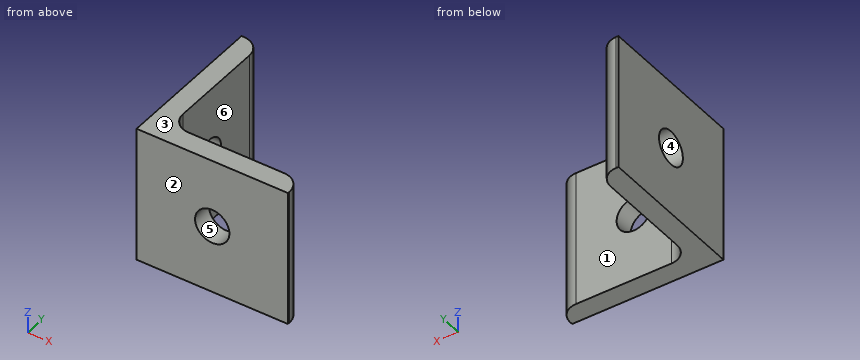
from build123d import *

# Parameters (mm, degrees)
BOSS_EXTRUDE1_DEPTH = 13.5
SKETCH4_R           = 3.4036
CUT_EXTRUDE3_DEPTH  = 10
SKETCH5_R           = 3.4036
CUT_EXTRUDE4_DEPTH  = 10


with BuildPart() as part:
    # Sketch1 → Boss-Extrude1 (new body, symmetric)
    with BuildSketch(Plane.XY):
        with BuildLine():
            Line((0, 0), (30, 0))
            Line((30, 0), (30, 0.5))
            ThreePointArc((30, 0.5), (28.974873734, 2.974873734), (26.5, 4))
            Line((26.5, 4), (7.5, 4))
            ThreePointArc((7.5, 4), (5.025126266, 5.025126266), (4, 7.5))
            Line((4, 7.5), (4, 26.5))
            ThreePointArc((4, 26.5), (2.974873734, 28.974873734), (0.5, 30))
            Line((0.5, 30), (0, 30))
            Line((0, 30), (0, 0))
        make_face()
    extrude(amount=BOSS_EXTRUDE1_DEPTH, both=True)

    # Sketch4 → Cut-Extrude3 (cut)
    with BuildSketch(Plane.ZY):
        with Locations((0, 15)):
            Circle(SKETCH4_R)
    extrude(amount=-CUT_EXTRUDE3_DEPTH, mode=Mode.SUBTRACT)

    # Sketch5 → Cut-Extrude4 (cut)
    with BuildSketch(Plane.XZ):
        with Locations((15, 0)):
            Circle(SKETCH5_R)
    extrude(amount=-CUT_EXTRUDE4_DEPTH, mode=Mode.SUBTRACT)


solid = part.part
Here's how the part is built. I have some questions about the finished solid (model axes, mm). Face numbers are marked on the shaded views. A direction names the side the tool comes from. Give positions to 0.01 mm unless a question says otherwise; leave off trailing zeros. Order: outer loops, then holes, each group sorted by start corner. A loop starts at its lowest first (then second) coordinate and runs counter-clockwise, first axis right, second up. Notation, with made-up numbers: (70.25, -2.75) -> (105.25, -2.75) arc R9 ccw to (105.25, 7.25) -> close; hole circle Ø6 at (46.5, 11.25). An arc over 180 degrees is marked (long way). Use a Markdown table: item, result. Add a question column.
Item 1: For the marked faces 1 and 2, which set-ups out of +Z, -Z, +X, -X, +Y, -Y let a thin tool reach every point of the face, with its end or its side?
Item 2: Imagine slicing it at D-D on z = -6.5. Please give me the cut outline in (x, y).
Item 3: Imagine slicing it at A-A on y = 15. Please give me the cut outline in (x, z).
Item 4: Imagine slicing it at C-C on z = 0. Please give me the cut outline in (x, y).
Item 5: Will these pins go through, and if not, where does the flat tip stop? pin 1 (12 mm diameter, centred on x = 22, z = 0.5, fed in from +Y); pin 2 (15 mm diameter, centred on y = 14, z = 5.5, fed in from +X).
Item 6: If we mould it in two halves opening along Z, with no side actions, what happens to the marked faces 3, 4, 5 and 6? For each: pulls with the +Z half, pulls with the -Z half, needs draft (parallel to the pull), parting line crosses it, or undercut.
Item 7: I need wall thicknesses on line 1 (Z direction, x = 15, y = 2.65); line 2 (X direction, y = 24.5, z = 12). Which ranges of each line are inside material? Lowest first, please.
Data:
| question | item | result |
|---|---|---|
| 1 | face 1 | +Z, -Z, +X, +Y |
| 1 | face 2 | +Z, -Z, +X, -X, -Y |
| 2 | outline | (0, 0) -> (30, 0) -> (30, 0.5) arc R3.5 ccw to (26.5, 4) -> (7.5, 4) arc R3.5 cw to (4, 7.5) -> (4, 26.5) arc R3.5 ccw to (0.5, 30) -> (0, 30) -> close |
| 3 | outline | (0, -13.5) -> (4, -13.5) -> (4, -3.4) -> (0, -3.4) -> close; (0, 3.4) -> (4, 3.4) -> (4, 13.5) -> (0, 13.5) -> close |
| 4 | outline | (0, 0) -> (11.6, 0) -> (11.6, 4) -> (7.5, 4) arc R3.5 cw to (4, 7.5) -> (4, 11.6) -> (0, 11.6) -> close; (0, 18.4) -> (4, 18.4) -> (4, 26.5) arc R3.5 ccw to (0.5, 30) -> (0, 30) -> close; (18.4, 0) -> (30, 0) -> (30, 0.5) arc R3.5 ccw to (26.5, 4) -> (18.4, 4) -> close |
| 5 | pin 1 | stops at y = 4 |
| 5 | pin 2 | stops at x = 4.15 |
| 6 | face 3 | pulls with the +Z half |
| 6 | face 4 | undercut |
| 6 | face 5 | undercut |
| 6 | face 6 | needs draft |
| 7 | line 1 | z = -13.5 to -3.4, 3.4 to 13.5 |
| 7 | line 2 | x = 0 to 4 |
